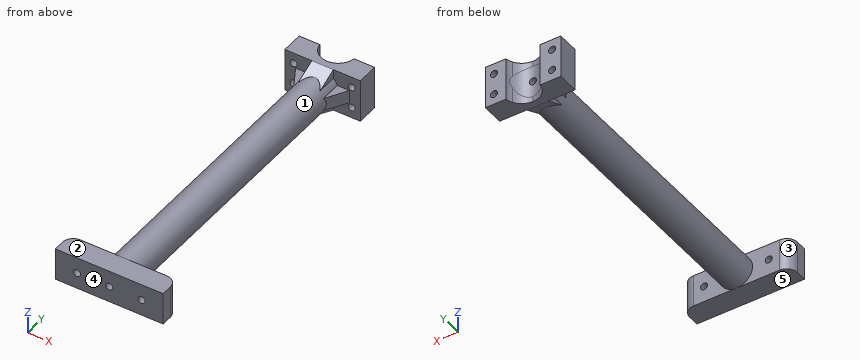
```python
from build123d import *

# Parameters (mm, degrees)
SKETCH_1_W               = 50
SKETCH_1_H               = 15
EXTRUDE_1_DEPTH          = 10
SKETCH_2_R               = 7.5
EXTRUDE_2_DEPTH          = 150
EXTRUDE_3_DEPTH          = 10
EXTRUDE_3_DEPTH_BACK     = 10
CUT_EXTRUDE_2_DEPTH      = 100
CUT_EXTRUDE_2_DEPTH_BACK = 100
SKETCH_5_R               = 1.65
CUT_EXTRUDE_3_DEPTH      = 10
FILLET_1_R               = 5
SKETCH_7_R               = 1.65
CUT_EXTRUDE_4_DEPTH      = 10
EXTRUDE_6_DEPTH          = 3
EXTRUDE_6_DEPTH_BACK     = 3
EXTRUDE_7_DEPTH          = 5
EXTRUDE_7_DEPTH_BACK     = 5


with BuildPart() as part:
    # 草图1 → 凸台-拉伸1 (new body)
    with BuildSketch(Plane(origin=(0, 0, 0), x_dir=(1, 0, 0), z_dir=(0, 1, 0))):
        Rectangle(SKETCH_1_W, SKETCH_1_H)
    extrude(amount=EXTRUDE_1_DEPTH)

    # 草图2 → 凸台-拉伸2 (add)
    with BuildSketch(Plane(origin=(0, 10, 0), x_dir=(1, 0, 0), z_dir=(0, 1, 0))):
        with Locations(Location((0, 0, 0), (0, 0, 270))):
            Circle(SKETCH_2_R)
    extrude(amount=EXTRUDE_2_DEPTH)

    # 草图3 → 凸台-拉伸3 (add, two sides: drawn at the far end of the back side and taken through both)
    with BuildSketch(Plane.XY.offset(-EXTRUDE_3_DEPTH_BACK)):
        with BuildLine():
            ThreePointArc((-10.246950766, 156), (-10.706300052, 157.4750962), (-10.95445115, 159))
            Line((-10.95445115, 159), (-17.5, 159))
            Line((-17.5, 159), (-17.5, 156))
            Line((-17.5, 156), (-10.246950766, 156))
        make_face()
        with BuildLine():
            ThreePointArc((-6.92820323, 156), (-7.582575695, 157.449598888), (-7.937253933, 159))
            Line((-7.937253933, 159), (-10.95445115, 159))
            ThreePointArc((-10.95445115, 159), (-10.706300052, 157.4750962), (-10.246950766, 156))
            Line((-10.246950766, 156), (-6.92820323, 156))
        make_face()
        with BuildLine():
            Line((10.95445115, 159), (7.937253933, 159))
            ThreePointArc((7.937253933, 159), (7.582575695, 157.449598888), (6.92820323, 156))
            Line((6.92820323, 156), (10.246950766, 156))
            ThreePointArc((10.246950766, 156), (10.706300052, 157.4750962), (10.95445115, 159))
        make_face()
        with BuildLine():
            ThreePointArc((6.92820323, 156), (4, 153.07179677), (0, 152))
            Line((0, 152), (0, 149))
            ThreePointArc((0, 149), (6.204836823, 150.917048938), (10.246950766, 156))
            Line((10.246950766, 156), (6.92820323, 156))
        make_face()
        with BuildLine():
            Line((0, 149), (0, 152))
            ThreePointArc((0, 152), (-4, 153.07179677), (-6.92820323, 156))
            Line((-6.92820323, 156), (-10.246950766, 156))
            ThreePointArc((-10.246950766, 156), (-6.204836823, 150.917048938), (0, 149))
        make_face()
        with BuildLine():
            Line((17.5, 159), (10.95445115, 159))
            ThreePointArc((10.95445115, 159), (10.706300052, 157.4750962), (10.246950766, 156))
            Line((10.246950766, 156), (17.5, 156))
            Line((17.5, 156), (17.5, 159))
        make_face()
        with BuildLine():
            Line((-17.5, 149), (0, 149))
            ThreePointArc((0, 149), (-6.204836823, 150.917048938), (-10.246950766, 156))
            Line((-10.246950766, 156), (-17.5, 156))
            Line((-17.5, 156), (-17.5, 149))
        make_face()
        with BuildLine():
            ThreePointArc((10.246950766, 156), (6.204836823, 150.917048938), (0, 149))
            Line((0, 149), (17.5, 149))
            Line((17.5, 149), (17.5, 156))
            Line((17.5, 156), (10.246950766, 156))
        make_face()
    extrude(amount=EXTRUDE_3_DEPTH + EXTRUDE_3_DEPTH_BACK)

    # 草图4 → 切除-拉伸2 (cut, two sides: drawn at the far end of the back side and taken through both)
    with BuildSketch(Plane.XY.offset(-CUT_EXTRUDE_2_DEPTH_BACK)):
        with BuildLine():
            Line((8, 160), (-8, 160))
            ThreePointArc((-8, 160), (-7.899200485, 158.734049095), (-7.599342077, 157.5))
            Line((-7.599342077, 157.5), (7.599342077, 157.5))
            ThreePointArc((7.599342077, 157.5), (7.899200485, 158.734049095), (8, 160))
        make_face()
        with BuildLine():
            Line((7.599342077, 157.5), (-7.599342077, 157.5))
            ThreePointArc((-7.599342077, 157.5), (0, 152), (7.599342077, 157.5))
        make_face()
    extrude(amount=CUT_EXTRUDE_2_DEPTH + CUT_EXTRUDE_2_DEPTH_BACK, mode=Mode.SUBTRACT)

    # 草图5 → 切除-拉伸3 (cut)
    with BuildSketch(Plane.XZ):
        with Locations(Location((0, 0, 0), (0, 0, 270))):
            Circle(SKETCH_5_R)
        with Locations(Location((-15, 0, 0), (0, 0, 270))):
            Circle(SKETCH_5_R)
        with Locations(Location((15, 0, 0), (0, 0, 270))):
            Circle(SKETCH_5_R)
    extrude(amount=-CUT_EXTRUDE_3_DEPTH, mode=Mode.SUBTRACT)

    # 草图6 → 切除-旋转1 (revolve, cut)
    with BuildSketch(Plane.XY, mode=Mode.PRIVATE) as cut_revolve_1_sk:
        Polygon((0, 10), (0, 20), (1.4, 20), (1.4, 15), (1.65, 10), align=None)
    revolve(cut_revolve_1_sk.sketch.rotate(Axis((0, 10, 0), (0, 1, 0)), 90), axis=Axis((0, 10, 0), (0, 1, 0)), mode=Mode.SUBTRACT)

    # 圆角1
    fillet_1_edges = [part.edges().sort_by_distance(p)[0] for p in [
        (-25, 10, 0),
        (25, 10, 0),
    ]]
    fillet(fillet_1_edges, radius=FILLET_1_R)

    # 草图9 → 切除-旋转2 (revolve, cut)
    with BuildSketch(Plane.XY, mode=Mode.PRIVATE) as cut_revolve_2_sk:
        Polygon((0, 152), (0, 153.423684137), (1.65, 153.423684137), (1.65, 149), (1.4, 144.61976638), (0, 144.61976638), (0, 149), align=None)
    revolve(cut_revolve_2_sk.sketch.rotate(Axis((0, 152, 0), (0, -1, 0)), 180), axis=Axis((0, 152, 0), (0, -1, 0)), mode=Mode.SUBTRACT)

    # 草图7 → 切除-拉伸4 (cut)
    with BuildSketch(Plane.XZ.offset(-149)):
        with Locations(Location((-13.5, 5, 0), (0, 0, 270))):
            Circle(SKETCH_7_R)
        with Locations(Location((-13.5, -5, 0), (0, 0, 270))):
            Circle(SKETCH_7_R)
        with Locations(Location((13.5, 5, 0), (0, 0, 270))):
            Circle(SKETCH_7_R)
        with Locations(Location((13.5, -5, 0), (0, 0, 270))):
            Circle(SKETCH_7_R)
    extrude(amount=-CUT_EXTRUDE_4_DEPTH, mode=Mode.SUBTRACT)

    # 草图10 → 凸台-拉伸6 (add, two sides: drawn at the far end of the back side and taken through both)
    with BuildSketch(Plane.XY.offset(-EXTRUDE_6_DEPTH_BACK)):
        Polygon((-12.5, 149), (-7.5, 149), (-7.5, 140.339745962), align=None)
        Polygon((0, 127.349364905), (0, 149), (-7.5, 149), (-7.5, 140.339745962), align=None)
        Polygon((7.5, 140.339745962), (7.5, 149), (0, 149), (0, 127.349364905), align=None)
        Polygon((7.5, 140.339745962), (12.5, 149), (7.5, 149), align=None)
    extrude(amount=EXTRUDE_6_DEPTH + EXTRUDE_6_DEPTH_BACK)

    # 草图11 → 凸台-拉伸7 (add, two sides: drawn at the far end of the back side and taken through both)
    with BuildSketch(Plane(origin=(0, 0, 0), x_dir=(0, 0, -1), z_dir=(1, 0, 0)).offset(-EXTRUDE_7_DEPTH_BACK)):
        Polygon((0, 149), (-10, 149), (0, 127.554930795), align=None)
        Polygon((10, 149), (0, 149), (0, 127.554930795), align=None)
    extrude(amount=EXTRUDE_7_DEPTH + EXTRUDE_7_DEPTH_BACK)


solid = part.part
```
Part model, mm, in its own coordinate system. Face numbers are marked on the shaded views. A direction names the side the tool comes from. Coordinates: 2 decimals unless noted, no trailing zeros. Loops run counter-clockwise (first coordinate to the right, second up) from the corner with the lowest first, then second, coordinate; pieces in that order, holes last. Notation, with made-up numbers: (4.5, 49.5) - (21.5, 49.5) arc R27 ccw to (21.5, 85.5) - close; hole circle Ø3 at (-36, -8.5). An arc over 180 degrees is marked (long way). Write item = value, one per line. Start each with the question number.
Item 1: Cut at A-A, the plane y = 16.5. Give the cut face in (x, z).
Item 2: Cut at C-C, the plane z = 0. State how many separate pieces and enclosed holes the cut face has, and give its area (3 significant figures).
Item 3: Cut at B-B, the plane y = 131. Give the cut face in (x, z), and give its area (3 significant figures).
Item 4: Flat gauge pins, fed straight in: pin 1 Ø2 at (x, z) = (0, 0) entering from -Y; pin 2 Ø5 at (y, z) = (145.5, 8) entering from -X; pin 3 Ø1.3 at (y, z) = (144, 7) entering from +X. Where does each tip first touch, or does it go through?
Item 5: 3-axis set-ups, long thin cutter, end or side, ignore diameter. For the marked faces 1, 2, 3, 4 and 5: which of +Z, -Z, +X, -X, +Y, -Y reach the whole face in a straight line?
Item 6: Wall check: L1, parallel to X at y = 151.5, z = -5; L2, parallel to Y at x = -16, z = -2; L3, parallel to Z at x = -13, y = 154. Give the ranges that are in metal, low to high. Write a range as from..to.
The answers:
q1.outline = circle Ø15 at (0, 0); hole circle Ø2.8 at (0, 0)
q2.separate_pieces = 3
q2.enclosed_holes = 0
q2.area = 2,740 mm2
q3.outline = circle Ø15 at (0, 0)
q3.area = 177 mm2
q4.pin_1 = 20
q4.pin_2 = -5.1
q4.pin_3 = 5
q5.face_1 = none
q5.face_2 = +Z, +X, -X, -Y
q5.face_3 = +Z, -Z, -X, +Y
q5.face_4 = +Z, -Z, +X, -X, -Y
q5.face_5 = -Z, +X, -X, -Y
q6.L1 = -17.5..-15.15, -11.85..11.85, 15.15..17.5
q6.L2 = 0..10, 149..159
q6.L3 = -10..-6.57, -3.43..3.43, 6.57..10
